```python
from build123d import *

# Parameters (mm, degrees)
F0_W      = 72
F0_H      = 10
F1_DEPTH  = 16
F3_DEPTH  = 25
F5_D      = 6
F5_DEPTH  = 10
F5_TIP    = 1.8025818571
F6_SIZE   = 0.5
F7_SIZE   = 5
F8_R      = 1
F10_DEPTH = 20


with BuildPart() as f1:
    # F0 (on Top) → F1 (new body)
    with BuildSketch(Plane.XY):
        Rectangle(F0_W, F0_H)
    extrude(amount=F1_DEPTH)

    # F2 (on face) → F3 (cut)
    with BuildSketch(Plane.XZ.offset(5)):
        Polygon((-36, 16), (-36, 4), (-14.5, 4), (-14.5, 6), (0.5, 6), (0.5, 16), align=None)
    extrude(amount=-F3_DEPTH, mode=Mode.SUBTRACT)

    # F5
    with Locations(Plane(origin=(0.5, 0, 0), x_dir=(0, -1, 0), z_dir=(-1, 0, 0))):
        with Locations((0, 11)):
            Hole(F5_D / 2, depth=F5_DEPTH)
            with Locations((0, 0, -(F5_DEPTH + F5_TIP / 2))):  # 118° drill point
                Cone(0, F5_D / 2, F5_TIP, mode=Mode.SUBTRACT)

    # F6
    f6_edges = [f1.edges().sort_by_distance(p)[0] for p in [
        (-36, 0, 4),
        (-36, -5, 2),
        (-36, 5, 2),
    ]]
    chamfer(f6_edges, length=F6_SIZE)

    # F7
    f7_edges = [f1.edges().sort_by_distance(p)[0] for p in [
        (36, 0, 16),
    ]]
    chamfer(f7_edges, length=F7_SIZE)

    # F8
    f8_edges = [f1.edges().sort_by_distance(p)[0] for p in [
        (15.75, -5, 16),
        (15.75, 5, 16),
    ]]
    fillet(f8_edges, radius=F8_R)

    # F9 (on Top) → F10 (cut)
    with BuildSketch(Plane.XY):
        with BuildLine():
            ThreePointArc((34.2449979984, 5), (36, 0), (34.2449979984, -5))
            Line((34.2449979984, -5), (37.1483493294, -5))
            Line((37.1483493294, -5), (37.1483493294, 5))
            Line((37.1483493294, 5), (34.2449979984, 5))
        make_face()
    extrude(amount=F10_DEPTH, mode=Mode.SUBTRACT)


solid = f1.part
```
The model under review builds one solid part; all positions refer to its coordinate system, in mm. A direction names the side the tool comes from. Coordinates: 2 decimals unless noted, no trailing zeros. Write each loop counter-clockwise with the first axis right and the second up, starting at its lowest first coordinate (ties: lowest second). Pieces come first, ordered by that corner, then holes. Notation, with made-up numbers: (48, 20.5) -> (93, 20.5) arc R23 ccw to (93, 44.5) -> close; hole circle Ø2 at (61, 76). An arc over 180 degrees is marked (long way). One line per item, written item: value. Start each with the question number.
Q1. To check wall thickness, follow probe 1 along Y at (x, z) = (8.5, 11); probe 2 along Z at (x, y) = (7, 0); probe 3 along Z at (x, y) = (-25, 2.25). State the ranges of each line that lie inside material, in increasing order.
Q2. The part is to be moulded in two halves that separate along Z. For faces 4 (the face through (7, 5, 6)), 5 (the face through (16, 0, 16)), 6 (the face through (11.99, -0.24, 10.54)), say which applies: +Z half, -Z half, draft (parallel to the pull), parting line (faces both ways), or undercut.
Q3. For faces 1 (the face through (5.57, -0.65, 8.07)), 2 (the face through (36, 0, 6)), 3 (the face through (0.5, -2.3, 8.7)), list the 3-axis set-ups (+Z, -Z, +X, -X, +Y, -Y) from which the entire face can be reached by the end or side of a thin tool; tool diameter is ignored.
Q4. Add section A-A, the plane x = -7. Give the boundary of the cut face in (y, z).
Q5. Clearance check with flat-ended pins moving along their axes: P1, Ø3, axis at y = -3.5, z = 14, coming from the -X side; P2, Ø4, axis at y = 3.5, z = 10.5, coming from the +X side; P3, Ø5, axis at x = -10.5, y = -2, coming from the +Z side. State where each tip first meets the part, or that it passes through.
Response:
1. probe 1: -5 to -3, 3 to 5
1. probe 2: 0 to 8, 14 to 16
1. probe 3: 0 to 4
2. face 4: draft
2. face 5: +Z half
2. face 6: undercut
3. face 1: -X
3. face 2: +Z, -Z, +X
3. face 3: +Z, -X, +Y, -Y
4. outline: (-5, 0) -> (5, 0) -> (5, 6) -> (-5, 6) -> close
5. P1: x = 0.5
5. P2: x = 35.86
5. P3: z = 6
